```python
from build123d import *

# Parameters (mm, degrees)
F0_W     = 12.7
F0_H     = 12.7
F1_DEPTH = 12.7
F2_W     = 1.5875
F2_H     = 6.35
F3_DEPTH = 12.7


with BuildPart() as f1:
    # F0 (on Top) → F1 (new body)
    with BuildSketch(Plane.XY):
        Rectangle(F0_W, F0_H)
    extrude(amount=F1_DEPTH)

    # F2 (on face) → F3 (cut, through all)
    with BuildSketch(Plane.XZ.offset(6.35)):
        with Locations((0, 3.175)):
            Rectangle(F2_W, F2_H)
    extrude(amount=-F3_DEPTH, mode=Mode.SUBTRACT)


solid = f1.part
```
The model under review builds one solid part; all positions refer to its coordinate system, in mm. A direction names the side the tool comes from. Round coordinates to 2 decimals unless told otherwise and drop trailing zeros. Write each loop counter-clockwise with the first axis right and the second up, starting at its lowest first coordinate (ties: lowest second). Pieces come first, ordered by that corner, then holes.
(1) Machinability: for faces 5 (the flat face through (0, -6.35, 8)), 6 (the flat face through (-0.794, 0, 3)), which of the approach directions +Z, -Z, +X, -X, +Y, -Y give a long, thin tool a straight path to every point of the face, cutting with its end or side? Answer none if there is none.
(2) Mouldability with a two-part tool opening along X and no side actions: class faces 1 (the flat face through (4, 0, 0)), 2 (the flat face through (0, 0, 6.35)), 3 (the flat face through (6.35, 0, 6)), 4 (the flat face through (-6.35, 0, 6)) as +X half, -X half, draft (parallel to the pull), parting line (faces both ways), or undercut.
(3) We need section B-B on y = 5.5. Give the boundary of the cut face in (x, z).
(4) We need section A-A on z = 2.75. Give the boundary of the cut face in (x, y).
(5) Wall thickness on L1, parallel to X at y = 3.5, z = 2.75; L2, parallel to Z at x = 0.75, y = 2.75: over which ranges is each line inside the solid? List them lowest first.
Findings below:
1. face 5: +Z, -Z, +X, -X, -Y
1. face 6: -Z, +Y, -Y
2. face 1: draft
2. face 2: undercut
2. face 3: +X half
2. face 4: -X half
3. outline: (-6.35, 0) - (-0.79, 0) - (-0.79, 6.35) - (0.79, 6.35) - (0.79, 0) - (6.35, 0) - (6.35, 12.7) - (-6.35, 12.7) - close
4. outline: (-6.35, -6.35) - (-0.79, -6.35) - (-0.79, 6.35) - (-6.35, 6.35) - close; (0.79, -6.35) - (6.35, -6.35) - (6.35, 6.35) - (0.79, 6.35) - close
5. L1: x = -6.35 to -0.79, 0.79 to 6.35
5. L2: z = 6.35 to 12.7
